Design review of the part built by this model. Coordinates are the model's own, in mm. A direction names the side the tool comes from. Give positions to 0.01 mm unless a question says otherwise; leave off trailing zeros. Write each loop counter-clockwise with the first axis right and the second up, starting at its lowest first coordinate (ties: lowest second). Pieces come first, ordered by that corner, then holes. Notation, with made-up numbers: (62.25, 38.5) -> (100.25, 38.5) arc R20 cw to (100.25, 54.5) -> close; hole circle Ø3 at (56.25, 65.5). An arc over 180 degrees is marked (long way). Use CSV: the item, a comma, the result in double quotes.
```python
from build123d import *

# Parameters (mm, degrees)
SKETCH1_R           = 0.635000006
BOSS_EXTRUDE1_DEPTH = 1.016
SKETCH2_W           = 17.907
SKETCH2_H           = 6.0198
BOSS_EXTRUDE2_DEPTH = 2.1082


with BuildPart() as part:
    # Sketch1 → Boss-Extrude1 (new body)
    with BuildSketch(Plane.XY):
        with BuildLine():
            Line((-7.4676, 7.4676), (7.4676, 7.4676))
            Line((7.4676, 7.4676), (7.4676, 2.0828))
            Line((7.4676, 2.0828), (8.808625011, 2.0828))
            ThreePointArc((8.808625011, 2.0828), (10.946108081, 0.126055131), (8.9535, -1.978035503))
            Line((8.9535, -1.978035503), (8.9535, -7.4676))
            Line((8.9535, -7.4676), (-8.9535, -7.4676))
            Line((-8.9535, -7.4676), (-8.9535, -1.978035503))
            ThreePointArc((-8.9535, -1.978035503), (-10.947109486, 0.019247939), (-9.022174989, 2.0828))
            Line((-9.022174989, 2.0828), (-7.4676, 2.0828))
            Line((-7.4676, 2.0828), (-7.4676, 7.4676))
        make_face()
        with Locations((-8.9154, 0.053607278)):
            Circle(SKETCH1_R, mode=Mode.SUBTRACT)
        with Locations((8.9154, 0.053607278)):
            Circle(SKETCH1_R, mode=Mode.SUBTRACT)
    extrude(amount=BOSS_EXTRUDE1_DEPTH)

    # Sketch2 → Boss-Extrude2 (add)
    with BuildSketch(Plane.XY.offset(1.016)):
        with Locations((0, -4.4577)):
            Rectangle(SKETCH2_W, SKETCH2_H)
    extrude(amount=BOSS_EXTRUDE2_DEPTH)


solid = part.part
```
(1) Take a section at D-D (z = 2.05). Write out the cut boundary in (x, y), then the cut area to 3 significant figures.
Established:
outline,"(-8.95, -7.47) -> (8.95, -7.47) -> (8.95, -1.45) -> (-8.95, -1.45) -> close"
area,"108 mm2"
(2) Clearance check with flat-ended pins moving along their axes: pin 1 (1.1 mm diameter, centred on y = 4.5, z = 0.5, fed in from +X); pin 2 (0.8 mm diameter, centred on x = 8, z = 0.5, fed in from +Y); pin 3 (0.6 mm diameter, centred on x = 2.5, z = 1.5, fed in from +Y); pin 4 (0.8 mm diameter, centred on x = 8.92, y = 0.05, fed in from -Z) (1 decimal). State where each tip first meets the part, or that it passes through.
Established:
pin 1,"stops at x = 7.47"
pin 2,"stops at y = 2.08"
pin 3,"stops at y = -1.45"
pin 4,"passes through"
(3) Take a section at B-B (x = 2.75). Write out the cut boundary in (y, z).
Established:
outline,"(-7.47, 0) -> (7.47, 0) -> (7.47, 1.02) -> (-1.45, 1.02) -> (-1.45, 3.12) -> (-7.47, 3.12) -> close"
(4) Take a section at C-C (y = 4). Write out the cut boundary in (x, z), then the cut area to 3 significant figures.
Established:
outline,"(-7.47, 0) -> (7.47, 0) -> (7.47, 1.02) -> (-7.47, 1.02) -> close"
area,"15.2 mm2"
(5) Take a section at A-A (z = 0.3). Write out the cut boundary in (x, y) (1 decimal), then the cut area to 3 significant figures.
Established:
outline,"(-9, -7.5) -> (9, -7.5) -> (9, -2) arc R2 ccw (long way) to (8.8, 2.1) -> (7.5, 2.1) -> (7.5, 7.5) -> (-7.5, 7.5) -> (-7.5, 2.1) -> (-9, 2.1) arc R2 ccw to (-9, -2) -> close; hole circle Ø1.3 at (-8.9, 0.1); hole circle Ø1.3 at (8.9, 0.1)"
area,"262 mm2"
(6) For line 1 along X through (y, z) = (-0.5, 0.9); line 2 along X through (y, z) = (-4, 1.35); line 3 along X through (y, z) = (6, 0.4), list the stretches that pass through material, from the lowest coordinate up. Write a range as [from, to].
Established:
line 1,"x = [-10.87, -9.23], [-8.6, 8.6], [9.23, 10.87]"
line 2,"x = [-8.95, 8.95]"
line 3,"x = [-7.47, 7.47]"
(7) Tool access review of faces 4 (the face through (-7.468, 4.7, 0.5)), 5 (the face through (0, -4, 3.124)): name each direction out of +Z, -Z, +X, -X, +Y, -Y from which nothing blocks a thin tool from reaching the whole face with its end or side.
Established:
face 4,"+Z, -Z, -X, +Y"
face 5,"+Z, +X, -X, +Y, -Y"
(8) Mouldability with a two-part tool opening along X and no side actions: class faces 1 (the face through (7.468, 4.8, 0.5)), 2 (the face through (9.5, -0.19, 0.5)), 3 (the face through (0, -1.448, 2)) as +X half, -X half, draft (parallel to the pull), parting line (faces both ways), or undercut.
Established:
face 1,"+X half"
face 2,"undercut"
face 3,"draft"
